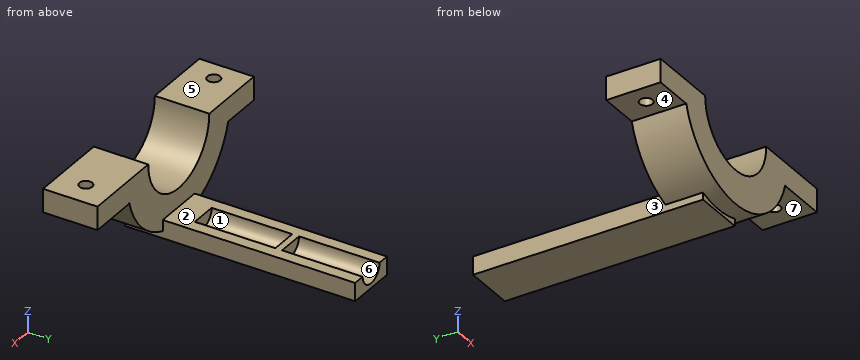
from build123d import *

# Parameters (mm, degrees)
SKETCH_1_W                = 48.51
SKETCH_1_H                = 34
SKETCH_1_W_2              = 28.51
SKETCH_1_H_2              = 14
EXTRUDE_1_DEPTH           = 12.25
SKETCH_2_R                = 1.91
CUT_EXTRUDE_1_DEPTH       = 33.05257439
SKETCH_4_W                = 13
SKETCH_4_H                = 13.91
EXTRUDE_1_2_DEPTH         = 74.82
SKETCH_5_W                = 13.91
SKETCH_5_H                = 16.23
EXTRUDE_2_DEPTH           = 15
SKETCH_7_R                = 24.5
SKETCH_7_R_2              = 14.5
EXTRUDE_2_2_DEPTH         = 16.23
SKETCH_12_R               = 1.9
CUT_EXTRUDE_4_DEPTH       = 97.312124675
EXTRUDE_3_DEPTH           = 10
EXTRUDE_3_DEPTH_BACK      = 8
SKETCH_13_W               = 13.91
SKETCH_13_H               = 16.23
SKETCH_14_R               = 1.9
CUT_EXTRUDE_5_DEPTH       = 103.744583434
SKETCH_16_W               = 90.709398763
SKETCH_16_H               = 28.955068616
CUT_EXTRUDE_7_DEPTH       = 111.229011154
SKETCH_18_W               = 13
SKETCH_18_H               = 93.080932143
CUT_EXTRUDE_10_DEPTH      = 27
CUT_EXTRUDE_11_DEPTH      = 57
CUT_EXTRUDE_11_DEPTH_BACK = 27
SKETCH_17_W               = 20.23049449
SKETCH_17_H               = 80.723570055
SKETCH_21_W               = 15.09856282
SKETCH_21_H               = 42.5
EXTRUDE_6_DEPTH           = 10
SKETCH_22_R               = 4.005
CUT_EXTRUDE_12_DEPTH      = 24
SKETCH_23_W               = 15.09856282
SKETCH_23_H               = 4.587452919
CUT_EXTRUDE_13_DEPTH      = 85.439664289
SKETCH_24_W               = 15.09856282
SKETCH_24_H               = 5.412547081
EXTRUDE_8_DEPTH           = 26
SKETCH_25_R               = 4.005
CUT_EXTRUDE_14_DEPTH      = 24


with BuildPart() as part:
    # 草圖1 → Extrude 1 (new body)
    with BuildSketch(Plane(origin=(0, 0, 0), x_dir=(1, 0, 0), z_dir=(0, 1, 0))):
        Rectangle(SKETCH_1_W, SKETCH_1_H)
        Rectangle(SKETCH_1_W_2, SKETCH_1_H_2, mode=Mode.SUBTRACT)
    extrude(amount=EXTRUDE_1_DEPTH)

    # 草圖2 → 除料-伸長1 (cut, through all)
    with BuildSketch(Plane(origin=(0, 12.25, 0), x_dir=(1, 0, 0), z_dir=(0, 1, 0))):
        with Locations(Location((-19.255, 0, 0), (0, 0, 270))):
            Circle(SKETCH_2_R)
        with Locations(Location((19.255, 0, 0), (0, 0, 270))):
            Circle(SKETCH_2_R)
    extrude(amount=-CUT_EXTRUDE_1_DEPTH, mode=Mode.SUBTRACT)

    # 草圖4 → Extrude 1 2 (add)
    with BuildSketch(Plane.XZ):
        with Locations((17.755, 0)):
            Rectangle(SKETCH_4_W, SKETCH_4_H)
    extrude(amount=EXTRUDE_1_2_DEPTH)

    # 草圖5 → Extrude 2 (add)
    with BuildSketch(Plane.ZY.offset(-11.255)):
        with Locations((0, -66.705)):
            Rectangle(SKETCH_5_W, SKETCH_5_H)
    extrude(amount=EXTRUDE_2_DEPTH)

    # 草圖7 → Extrude 2 2 (add)
    with BuildSketch(Plane(origin=(3.626674765, -74.82, 0), x_dir=(1, 0, 0), z_dir=(0, -1, 0))):
        with Locations((-30.978154344, 0)):
            Circle(SKETCH_7_R)
        with Locations((-30.978154344, 0)):
            Circle(SKETCH_7_R_2, mode=Mode.SUBTRACT)
    extrude(amount=-EXTRUDE_2_2_DEPTH)

    # 草圖12 → 除料-伸長4 (cut, through all)
    with BuildSketch(Plane(origin=(0, 0, -6.955), x_dir=(-1, 0, 0), z_dir=(0, 0, -1))):
        with Locations((-3.856713649, -66.705)):
            Circle(SKETCH_12_R)
    extrude(amount=-CUT_EXTRUDE_4_DEPTH, mode=Mode.SUBTRACT)

    # 草圖13 → 填料-伸長3 (add, two sides: drawn at the far end of the back side and taken through both)
    with BuildSketch(Plane(origin=(-55, 0, 0), x_dir=(0, 0, -1), z_dir=(1, 0, 0)).offset(-EXTRUDE_3_DEPTH_BACK)):
        with Locations((0, -66.705)):
            Rectangle(SKETCH_13_W, SKETCH_13_H)
    extrude(amount=EXTRUDE_3_DEPTH + EXTRUDE_3_DEPTH_BACK)

    # 草圖14 → 除料-伸長5 (cut, through all)
    with BuildSketch(Plane(origin=(0, 0, -6.955), x_dir=(-1, 0, 0), z_dir=(0, 0, -1))):
        with Locations((56.908040017, -66.705)):
            Circle(SKETCH_14_R)
    extrude(amount=-CUT_EXTRUDE_5_DEPTH, mode=Mode.SUBTRACT)

    # 草圖16 → 除料-伸長7 (cut, through all)
    with BuildSketch(Plane(origin=(0, 12.25, 0), x_dir=(1, 0, 0), z_dir=(0, 1, 0))):
        with Locations((-17.645300619, -14.477534308)):
            Rectangle(SKETCH_16_W, SKETCH_16_H)
    extrude(amount=-CUT_EXTRUDE_7_DEPTH, mode=Mode.SUBTRACT)

    # 草圖18 → 除料-伸長10 (cut)
    with BuildSketch(Plane.XY):
        with Locations((17.755, -28.279533929)):
            Rectangle(SKETCH_18_W, SKETCH_18_H)
    extrude(amount=-CUT_EXTRUDE_10_DEPTH, mode=Mode.SUBTRACT)


with BuildPart() as cut_extrude_10_piece_1:
    # of the separate pieces the step leaves, piece 1, a body of its own (cut_extrude_10_pieces)
    add(part.part.solids().sort_by_distance((11.255, -58.59, -6.955))[0])

    # 草圖21 → 填料-伸長6 (add)
    with BuildSketch(Plane.XY.offset(-30)):
        with Locations((-27.29428141, -48.519427919)):
            Rectangle(SKETCH_21_W, SKETCH_21_H)
    extrude(amount=EXTRUDE_6_DEPTH)

    # 草圖22 → 除料-伸長12 (cut)
    with BuildSketch(Plane(origin=(0, -27.269427919, 0), x_dir=(1, 0, 0), z_dir=(0, 1, 0))):
        with Locations((-27.29428141, 20)):
            Circle(SKETCH_22_R)
    extrude(amount=-CUT_EXTRUDE_12_DEPTH, mode=Mode.SUBTRACT)

    # 草圖23 → 除料-伸長13 (cut, through all)
    with BuildSketch(Plane(origin=(0, -27.269427919, 0), x_dir=(1, 0, 0), z_dir=(0, 1, 0))):
        with Locations((-27.29428141, 27.706273541)):
            Rectangle(SKETCH_23_W, SKETCH_23_H)
    extrude(amount=-CUT_EXTRUDE_13_DEPTH, mode=Mode.SUBTRACT)

    # 草圖24 → 填料-伸長8 (add)
    with BuildSketch(Plane(origin=(0, -27.269427919, 0), x_dir=(1, 0, 0), z_dir=(0, 1, 0))):
        with Locations((-27.29428141, 22.70627354)):
            Rectangle(SKETCH_24_W, SKETCH_24_H)
    extrude(amount=EXTRUDE_8_DEPTH)

    # 草圖25 → 除料-伸長14 (cut)
    with BuildSketch(Plane(origin=(0, -1.269427919, 0), x_dir=(1, 0, 0), z_dir=(0, 1, 0))):
        with Locations((-27.29428141, 20)):
            Circle(SKETCH_25_R)
    extrude(amount=-CUT_EXTRUDE_14_DEPTH, mode=Mode.SUBTRACT)


with BuildPart() as cut_extrude_10_piece_2:
    # of the separate pieces the step leaves, piece 2, a body of its own (cut_extrude_10_pieces)
    add(part.part.solids().sort_by_distance((-17.345, 0, 0))[0])

    # 草圖17 → 除料-伸長11 (cut, two sides: drawn at the far end of the back side and taken through both)
    with BuildSketch(Plane.ZY.offset(-11.255).offset(-CUT_EXTRUDE_11_DEPTH_BACK)):
        with Locations((-10.115247245, -18.228214973)):
            Rectangle(SKETCH_17_W, SKETCH_17_H)
    extrude(amount=CUT_EXTRUDE_11_DEPTH + CUT_EXTRUDE_11_DEPTH_BACK, mode=Mode.SUBTRACT)


solid = cut_extrude_10_piece_1.part
The model under review builds one solid part; all positions refer to its coordinate system, in mm. Face numbers are marked on the shaded views. A direction names the side the tool comes from. Give positions to 0.01 mm unless a question says otherwise; leave off trailing zeros. Write each loop counter-clockwise with the first axis right and the second up, starting at its lowest first coordinate (ties: lowest second). Pieces come first, ordered by that corner, then holes. Notation, with made-up numbers: M -24,-20.75 L 34,-20.75 A23 ccw 34,-2.75 Z; hole C 76.5,-21 d11. An arc over 180 degrees is marked long. One line per question, with ' | ' between items. Start each with the question number.
Item 1: Wall thickness on line 1 (X direction, y = -67, z = -5.5) (3 decimals); line 2 (X direction, y = -47.5, z = -22.75) (3 decimals); line 3 (X direction, y = -54.5, z = -23.25) (3 decimals): over which ranges is each line inside the solid? List them lowest first. Write a range as from..to.
Item 2: We need section C-C on y = -38. Write out the cut boundary in (x, z) (3 decimals), plus the area to 3 significant figures.
Item 3: For pin 1 (6 mm diameter, centred on y = -42, z = -23.5, fed in from -X); pin 2 (13.5 mm diameter, centred on x = -59, y = -62.5, fed in from -Z) (3 decimals); pin 3 (10 mm diameter, centred on x = -36.5, y = -33.5, fed in from +Z), all flat-tipped, find the tip position at first contact; note any pin that passes through.
Item 4: For the marked faces 4, 5, 6 and 7, list the 3-axis set-ups (+Z, -Z, +X, -X, +Y, -Y) from which the entire face can be reached by the end or side of a thin tool; tool diameter is ignored.
Item 5: We need section D-D on z = -10.25. Write out the cut boundary in (x, y).
Item 6: We need section B-B on x = -30. Write out the cut boundary in (y, z).
Item 7: Draft analysis for pull direction X (two halves, no side actions). For the marked faces 1, 2 and 3, state which applies: released by +X, released by -X, zero draft, split by the parting line, or undercut.
Item 8: We need section A-A on z = -5.25. Write out the cut boundary in (x, y) (3 decimals).
Results found:
1) line 1: x = -63..-58.785, -55.031..-40.768, -13.935..1.98, 5.734..11.255 | line 2: x = -34.844..-30.206, -24.383..-19.745 | line 3: x = -34.844..-19.745
2) outline: M -34.844,-25.413 L -19.745,-25.413 L -19.745,-20 L -23.289,-20 A4.005 cw -31.299,-20 L -34.844,-20 Z | area: 56.5 mm2
3) pin 1: stops at x = -34.84 | pin 2: stops at z = -6.955 | pin 3: stops at z = -20
4) face 4: -Z, -X, +Y, -Y | face 5: +Z, +X, -X, +Y, -Y | face 6: +Z, +Y | face 7: -Z, +X, +Y, -Y
5) outline: M -49.6,-74.82 L -37.61,-74.82 L -37.61,-58.59 L -49.6,-58.59 Z; M -17.1,-74.82 L -5.1,-74.82 L -5.1,-58.59 L -17.1,-58.59 Z
6) outline: M -74.82,-24.36 L -69.77,-24.36 L -69.77,-25.41 L -1.27,-25.41 L -1.27,-22.95 L -25.27,-22.95 L -25.27,-20 L -27.27,-20 L -27.27,-22.95 L -51.27,-22.95 L -51.27,-20 L -58.59,-20 L -58.59,-14.26 L -74.82,-14.26 Z
7) face 1: undercut | face 2: zero draft | face 3: released by -X
8) outline: M -63,-74.82 L -40.868,-74.82 L -40.868,-58.59 L -63,-58.59 Z; M -13.835,-74.82 L 11.255,-74.82 L 11.255,-58.59 L -13.835,-58.59 Z; hole C -56.908,-66.705 d3.8; hole C 3.857,-66.705 d3.8
